from build123d import *
from build123d.topology import SkipClean

# Parameters (mm, degrees)
SKETCH1_W                       = 80
SKETCH1_H                       = 12
BOSS_EXTRUDE1_DEPTH             = 2
CUT_REVOLVE1_ANGLE              = 180
FILLET2_R                       = 4
BOSS_EXTRUDE2_REACH             = 42.645
SKETCH6_R                       = 17
BOSS_EXTRUDE2_DIRECTION_2_DEPTH = 2
SKETCH7_R                       = 2.5
CUT_EXTRUDE3_DEPTH              = 3
CIRPATTERN1_COUNT               = 6
FILLET3_R                       = 1
CUT_EXTRUDE4_REACH              = 61.783
SKETCH8_R                       = 1.5


with BuildPart() as part:
    # Sketch1 → Boss-Extrude1 (new, symmetric)
    with BuildSketch(Plane.XY):
        Rectangle(SKETCH1_W, SKETCH1_H)
    extrude(amount=BOSS_EXTRUDE1_DEPTH, both=True)

    # Sketch3 → Cut-Revolve1 (revolve, cut)
    with SkipClean():  # the faces are left unmerged after this step: merging them gives an invalid solid
        with BuildSketch(Plane.XY.offset(-2)):
            with BuildLine():
                ThreePointArc((37.75, 0), (35, 2.75), (32.25, 0))
                Line((32.25, 0), (37.75, 0))
            make_face()
            with BuildLine():
                Line((37.75, 0), (32.25, 0))
                ThreePointArc((32.25, 0), (35, -2.75), (37.75, 0))
            make_face()
        revolve(axis=Axis((32.25, 0, -2), (1, 0, 0)), revolution_arc=CUT_REVOLVE1_ANGLE, mode=Mode.SUBTRACT)

    # Fillet2
    fillet2_edges = [part.edges().sort_by_distance(p)[0] for p in [
        (40, -6, 0),
        (40, 6, 0),
    ]]
    fillet(fillet2_edges, radius=FILLET2_R)

    # Boss-Extrude2: up to this face of the body (flat: up to its plane)
    boss_extrude2_end = Plane(part.part.faces().sort_by_distance((-1.183693998, 0, -2))[0])
    # Sketch6 → Boss-Extrude2 (add, up to the picked face)
    with BuildSketch(Plane.XY.offset(2), mode=Mode.PRIVATE) as boss_extrude2_sk1:
        with Locations(Location((-40, 0, 0), (0, 0, 20.667316494))):
            Circle(SKETCH6_R)
    boss_extrude2_tool1 = split(extrude(boss_extrude2_sk1.sketch, amount=-BOSS_EXTRUDE2_REACH, mode=Mode.PRIVATE), bisect_by=boss_extrude2_end, keep=Keep.BOTH, mode=Mode.PRIVATE)
    add(boss_extrude2_tool1.solids().sort_by(Axis((-40, 0, 2), (0, 0, -1)))[0])

    # Sketch6 → Boss-Extrude2 direction 2 (add)
    with BuildSketch(Plane.XY.offset(2)):
        with Locations(Location((-40, 0, 0), (0, 0, 20.667316494))):
            Circle(SKETCH6_R)
    extrude(amount=BOSS_EXTRUDE2_DIRECTION_2_DEPTH)

    # Sketch7 → Cut-Extrude3 (cut)
    with BuildSketch(Plane(origin=(0, 0, -2), x_dir=(-1, 0, 0), z_dir=(0, 0, -1))):
        with BuildLine():
            Line((41.148365434, 4.169758006), (40, 4.325))
            ThreePointArc((40, 4.325), (35.675, 0), (40, -4.325))
            Line((40, -4.325), (41.148365434, -4.169758006))
            ThreePointArc((41.148365434, -4.169758006), (43.440371019, -2.620967808), (44.325, 0))
            ThreePointArc((44.325, 0), (43.440371019, 2.620967808), (41.148365434, 4.169758006))
        make_face()
        with BuildLine():
            Line((53.5, 2.5), (41.148365434, 4.169758006))
            ThreePointArc((41.148365434, 4.169758006), (43.440371019, 2.620967808), (44.325, 0))
            ThreePointArc((44.325, 0), (43.440371019, -2.620967808), (41.148365434, -4.169758006))
            Line((41.148365434, -4.169758006), (53.5, -2.5))
            ThreePointArc((53.5, -2.5), (51, 0), (53.5, 2.5))
        make_face()
        with Locations((53.5, 0)):
            Circle(SKETCH7_R)
    cut_extrude3 = extrude(amount=-CUT_EXTRUDE3_DEPTH, mode=Mode.SUBTRACT)

    # CirPattern1: Cut-Extrude3 ×6 about axis
    cirpattern1_axis = Axis((-40, 0, 0), (0, 0, 1))
    for i in range(1, CIRPATTERN1_COUNT):
        add(cut_extrude3.rotate(cirpattern1_axis, i * 360 / CIRPATTERN1_COUNT), mode=Mode.SUBTRACT)

    # Fillet3
    fillet3_edges = [part.edges().sort_by_distance(p)[0] for p in [
        (-46.069873399, 3.504443041, -0.5),
        (-40, 7.008886081, -0.5),
        (-33.930126601, 3.504443041, -0.5),
        (-33.930126601, -3.504443041, -0.5),
        (-40, -7.008886081, -0.5),
        (-46.069873399, -3.504443041, -0.5),
    ]]
    fillet(fillet3_edges, radius=FILLET3_R)

    # Sketch8 → Cut-Extrude4 (cut, up to next)
    with BuildSketch(Plane.XY.offset(4), mode=Mode.PRIVATE) as cut_extrude4_sk1:
        with Locations((-40, 0)):
            Circle(SKETCH8_R)
    cut_extrude4_tool1 = extrude(cut_extrude4_sk1.sketch, amount=-CUT_EXTRUDE4_REACH, mode=Mode.PRIVATE) & part.part
    add(cut_extrude4_tool1.solids().sort_by_distance((-40, 0, 4))[0], mode=Mode.SUBTRACT)


solid = part.part
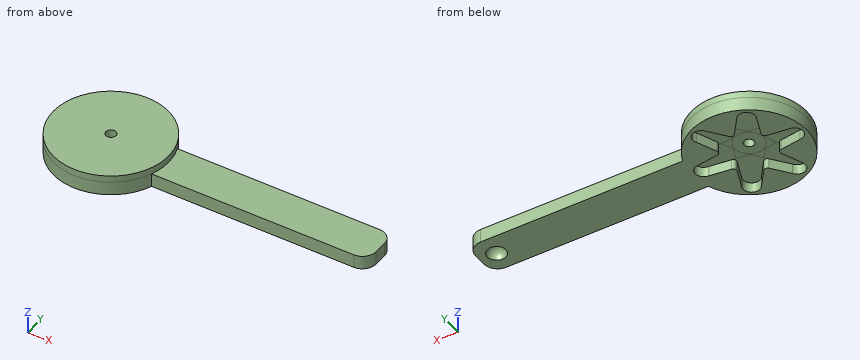
Verification items for the finished model (mm, model axes). Coordinates: 2 decimals unless noted, no trailing zeros. Loops run counter-clockwise (first coordinate to the right, second up) from the corner with the lowest first, then second, coordinate; pieces in that order, holes last. Notation, with made-up numbers: (-17.75, 44.25) -> (-1.75, 44.25) arc R23 cw to (-1.75, 66.25) -> close; hole circle Ø8 at (41.5, 47). An arc over 180 degrees is marked (long way). Answer as a JSON object with one key per item and string values. Group by question number.
Item 1: Depth check by flat-ended pin: pin 1 (9 mm diameter, centred on x = -29, y = 1, fed in from -Z); pin 2 (13 mm diameter, centred on x = -7, y = -0.5, fed in from +Z); pin 3 (0.8 mm diameter, centred on x = -36.5, y = -3, fed in from -Z); pin 4 (2 mm diameter, centred on x = 12, z = 0.5, fed in from -Y). Enter the tip coordinate at first touch or a pass-through.
Item 2: Sectioned sample at A-A on x = -15. Record the boundary of the cut face in (y, z).
Item 3: Scan lines: probe 1 along Y at (x, z) = (-40, 3.15); probe 2 along Y at (x, z) = (-47, -0.4); probe 3 along X at (y, z) = (-10, -0.55). Record each from-to range of solid material in increasing order.
Evaluation:
{
 "1": {"pin 1": "stops at z = -2", "pin 2": "stops at z = 2", "pin 3": "stops at z = 1", "pin 4": "stops at y = -6"},
 "2": {"outline": "(-6, -2) -> (6, -2) -> (6, 2) -> (-6, 2) -> close"},
 "3": {"probe 1": "y = -17 to -1.5, 1.5 to 17", "probe 2": "y = -15.49 to -14.18, -5.77 to -3.45, 3.45 to 5.77, 14.18 to 15.49", "probe 3": "x = -53.75 to -48.73, -42.31 to -37.69, -31.27 to -26.25"}
}
